Read the model definition and answer for the solid it produces. Units are mm, in the model's axes. A direction names the side the tool comes from. Coordinates: 2 decimals unless noted, no trailing zeros. Write each loop counter-clockwise with the first axis right and the second up, starting at its lowest first coordinate (ties: lowest second). Pieces come first, ordered by that corner, then holes. Notation, with made-up numbers: (41.25, 29.25) -> (53.25, 29.25) arc R28 cw to (53.25, 60.25) -> close; hole circle Ø6 at (75.5, -27). An arc over 180 degrees is marked (long way). Return JSON: item names as keys, results as strings.
from build123d import *

# Parameters (mm, degrees)
SKETCH1_R           = 3
BOSS_EXTRUDE1_DEPTH = 22
BOSS_EXTRUDE2_DEPTH = 3.95


with BuildPart() as part:
    # Sketch1 → Boss-Extrude1 (new body)
    with BuildSketch(Plane.XY):
        Circle(SKETCH1_R)
    extrude(amount=BOSS_EXTRUDE1_DEPTH)

    # Sketch2 → Boss-Extrude2 (add, symmetric)
    with BuildSketch(Plane(origin=(0, 0, 0), x_dir=(1, 0, 0), z_dir=(0, 1, 0))):
        Polygon((-5.55, -21), (-8.25, -18.3), (-8.25, -16.5), (-4, -16.5), (-4, -15), (4, -15), (4, -16.5), (8.25, -16.5), (8.25, -18.3), (5.55, -21), align=None)
    extrude(amount=BOSS_EXTRUDE2_DEPTH, both=True)


solid = part.part
1. The part is cut by section B-B (y = 0). Determine the outline of the cut face in (x, z).
Taken from the geometry:
{"outline": "(-8.25, 16.5) -> (-4, 16.5) -> (-4, 15) -> (-3, 15) -> (-3, 0) -> (3, 0) -> (3, 15) -> (4, 15) -> (4, 16.5) -> (8.25, 16.5) -> (8.25, 18.3) -> (5.55, 21) -> (3, 21) -> (3, 22) -> (-3, 22) -> (-3, 21) -> (-5.55, 21) -> (-8.25, 18.3) -> close"}
2. Consider L1, parallel to Z at x = -4.5, y = 1; L2, parallel to Z at x = 3.5, y = 1.5; L3, parallel to X at y = 3.5, z = 16. Determine where each line is inside the solid, lowest interval first.
Taken from the geometry:
{"L1": "z = 16.5 to 21", "L2": "z = 15 to 21", "L3": "x = -4 to 4"}
3. A tool of negligible diameter and unlimited length cuts with its end or side. For faces 1 (the face through (-3, 0, 7)), 2 (the face through (4, 0, 16)), 3 (the face through (-4, 0, 16)), from which of +Z, -Z, +X, -X, +Y, -Y can it reach the whole face along a straight path? Write none if from no direction.
Taken from the geometry:
{"face 1": "-Z", "face 2": "-Z, +X, +Y, -Y", "face 3": "-Z, -X, +Y, -Y"}
4. The part is cut by section A-A (x = 0). Determine the outline of the cut face in (y, z).
Taken from the geometry:
{"outline": "(-3.95, 15) -> (-3, 15) -> (-3, 0) -> (3, 0) -> (3, 15) -> (3.95, 15) -> (3.95, 21) -> (3, 21) -> (3, 22) -> (-3, 22) -> (-3, 21) -> (-3.95, 21) -> close"}
5. Flat-ended cylindrical pins translate along their axes: pin 1 Ø1.5 at (x, y) = (-6, -0.5) entering from +Z; pin 2 Ø2 at (x, y) = (-6.5, 0.5) entering from -Z; pin 3 Ø1.5 at (y, z) = (2.5, 14) entering from +X. Find the tip coordinate at first contact, or state that the pin passes through.
Taken from the geometry:
{"pin 1": "stops at z = 21", "pin 2": "stops at z = 16.5", "pin 3": "stops at x = 2.44"}
6. The part is cut by section D-D (x = -2). Determine the outline of the cut face in (y, z), then the cut area to 3 significant figures.
Taken from the geometry:
{"outline": "(-3.95, 15) -> (-2.24, 15) -> (-2.24, 0) -> (2.24, 0) -> (2.24, 15) -> (3.95, 15) -> (3.95, 21) -> (2.24, 21) -> (2.24, 22) -> (-2.24, 22) -> (-2.24, 21) -> (-3.95, 21) -> close", "area": "119 mm2"}
7. The part is cut by section C-C (z = 10.25). Determine the outline of the cut face in (x, y).
Taken from the geometry:
{"outline": "circle Ø6 at (0, 0)"}
